Source: CAD feature listing. Evaluate the final solid. Frame: model axes, mm. A direction names the side the tool comes from. Round coordinates to 2 decimals unless told otherwise and drop trailing zeros. Order: outer loops, then holes, each group sorted by start corner. A loop starts at its lowest first (then second) coordinate and runs counter-clockwise, first axis right, second up. Notation, with made-up numbers: (81, 35) - (137, 35) arc R13 cw to (137, 56) - close; hole circle Ø11 at (49, 85.25). An arc over 180 degrees is marked (long way). Use one line per item in the form item = value. Start each with the question number.
Q1. Set-up query: faces 4 (the flat face through (0, -21, 33)), 5 (the flat face through (-17, 0, -17)), 6 (the flat face through (-15, -19.05, -32)). Return all of +Z, -Z, +X, -X, +Y, -Y with unobstructed straight access to the full face (end or side cutting, diameter ignored); none if empty.
Q2. Pin query (flat end, axial travel): pin 1 Ø5 at (x, y) = (29, -10) entering from +Z; pin 2 Ø5 at (y, z) = (-7, -22) entering from +X; pin 3 Ø3 at (x, z) = (27.5, -27.5) entering from -Y; pin 4 Ø23 at (x, z) = (0, 0) entering from -Y. Return the tip coordinate at first contact, or that it passes through.
Q3. Cut plane D-D, the plane x = 30.5. Return the cut outline in (y, z).
Q4. Cut plane B-B, the plane y = -31. Return the cut outline in (x, z), and give its area (3 significant figures).
Q5. Ray query, line 1 (Y direction, x = -20, z = -44.5); line 2 (X direction, y = -28.5, z = -8.5); line 3 (X direction, y = -43, z = -4). Return the intervals inside material, ascending. Write a range as [from, to].
Q6. Cut plane C-C, the plane z = 52.5. Return the cut outline in (x, y).
Q7. Cut plane A-A, the plane x = -28.5. Return the cut outline in (y, z), and give its area (3 significant figures).
Q8. Draft query along X for faces 1 (the cylindrical face through (-13.89, -27.3, -13)), 2 (the flat face through (65, -9, 0)), 3 (the cylindrical face through (-47.74, -9.39, -50.99)). Return one class per face: released by +X, released by -X, zero draft, split by the parting line, or undercut.
from build123d import *

# Parameters (mm, degrees)
F1_ANGLE = 270
F3_DEPTH = 25.4
F5_DEPTH = 76.2


with BuildPart() as f1:
    # F0 (on Top) → F1 (revolve)
    with BuildSketch(Plane.XY):
        Polygon((69.85, 0), (0, 0), (0, -53.848), (35.052, -53.848), (35.052, -19.05), (69.85, -19.05), align=None)
    revolve(axis=Axis((0, -26.924, 0), (0, 1, 0)), revolution_arc=F1_ANGLE)

    # F2 (on face) → F3 (cut)
    with BuildSketch(Plane(origin=(0, 0, 0), x_dir=(-1, 0, 0), z_dir=(0, 1, 0))):
        with BuildLine():
            ThreePointArc((-60.198, 0), (-58.2037429965, -4.6206063399), (-53.4735896226, -6.3389523479))
            ThreePointArc((-53.4735896226, -6.3389523479), (-53.7543159104, -3.175), (-53.848, 0))
            Line((-53.848, 0), (-60.198, 0))
        make_face()
        with BuildLine():
            ThreePointArc((-53.848, 0), (-53.7543159104, -3.175), (-53.4735896226, -6.3389523479))
            ThreePointArc((-53.4735896226, -6.3389523479), (-49.2273936601, -4.3557429965), (-47.498, 0))
            Line((-47.498, 0), (-53.848, 0))
        make_face()
    extrude(amount=-F3_DEPTH, mode=Mode.SUBTRACT)

    # F4 (on face) → F5 (cut)
    with BuildSketch(Plane.XZ.offset(53.848)):
        with BuildLine():
            ThreePointArc((0, 19.0246), (-13.4524236694, -13.4524236694), (19.0246, 0))
            Line((19.0246, 0), (0, 0))
            Line((0, 0), (0, 19.0246))
        make_face()
    extrude(amount=-F5_DEPTH, mode=Mode.SUBTRACT)


solid = f1.part
Completed:
q1.face_4 = +Z, +X, +Y, -Y
q1.face_5 = +Z, -Z, +X, -X, +Y
q1.face_6 = -Y
q2.pin_1 = 0
q2.pin_2 = 67.07
q2.pin_3 = -19.05
q2.pin_4 = through
q3.outline = (-53.85, -17.27) - (-19.05, -17.27) - (-19.05, -62.84) - (0, -62.84) - (0, 0) - (-53.85, 0) - close
q4.outline = (0, 19.02) - (0, 35.05) arc R35.05 ccw (long way) to (35.05, 0) - (19.02, 0) arc R19.02 cw (long way) to start
q4.area = 2,040 mm2
q5.line_1 = [-19.05, 0]
q5.line_2 = [-34.01, -17.02], [17.02, 34.01]
q5.line_3 = [-34.82, -18.6], [18.6, 34.82]
q6.outline = (-46.07, -19.05) - (0, -19.05) - (0, 0) - (-46.07, 0) - close
q7.outline = (-53.85, -20.41) - (-19.05, -20.41) - (-19.05, -63.77) - (0, -63.77) - (0, 63.77) - (-19.05, 63.77) - (-19.05, 20.41) - (-53.85, 20.41) - close
q7.area = 3,850 mm2
q8.face_1 = undercut
q8.face_2 = zero draft
q8.face_3 = split by the parting line
